Source: CAD feature listing. Evaluate the final solid. Frame: model axes, mm. Face numbers are marked on the shaded views. A direction names the side the tool comes from. Give positions to 0.01 mm unless a question says otherwise; leave off trailing zeros. Order: outer loops, then holes, each group sorted by start corner. A loop starts at its lowest first (then second) coordinate and runs counter-clockwise, first axis right, second up. Notation, with made-up numbers: M 28.25,64.25 L 32.25,64.25 A32 ccw 32.25,99.25 Z; hole C 1.25,15.25 d2. An arc over 180 degrees is marked long. Use CSV: the item, a comma, the result in double quotes. Start each with the question number.
Item 1: Section query A-A on y = 60. Count the separate pieces of the cut face and the enclosed holes in it, and give its area (3 significant figures).
Item 2: Section query B-B on z = 3.5. Return loops of the section in (x, y), and give its area (3 significant figures).
Item 3: First-contact query: pin 1 (10 mm diameter, centred on x = -232.5, z = 23, fed in from -Y); pin 2 (17 mm diameter, centred on x = -6.5, z = 10, fed in from -Y). Flat tips, straight axial feed; report the tip coordinate or a pass-through.
Item 4: Pull-direction query (Z, two-part tool) for the marked faces 3, 4, 5 and 6; classes: +Z half, -Z half, draft (parallel to the pull), parting line (faces both ways), or undercut.
Item 5: Ray query, probe 1 along X at (y, z) = (44.5, 28); probe 2 along X at (y, z) = (75, 3.5); probe 3 along X at (y, z) = (66, 84). Return the intervals inside material, ascending. Write a range as from..to.
Item 6: Access query for the marked faces 1 and 2. Directions: +Z, -Z, +X, -X, +Y, -Y. A direction counts if a zero-diameter tool reaches every point of the face in a straight line with its end or side. Return the directions, or none.
Item 7: Section query D-D on x = -157. Return loops of the section in (y, z).
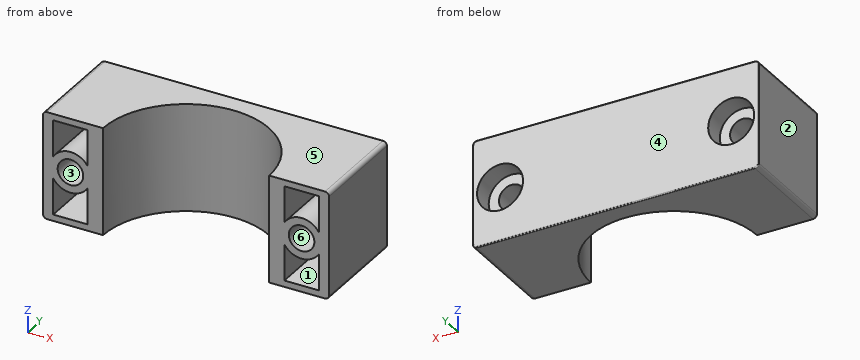
Autodesk Inventor part; units mm, degrees
ref_plane "YZ Plane" through (0, 0, 0) normal (1, 0, 0) x (0, 1, 0)
ref_plane "XZ Plane" through (0, 0, 0) normal (0, 1, 0) x (-1, 0, 0)
ref_plane "XY Plane" through (0, 0, 0) normal (0, 0, 1) x (1, 0, 0)
sketch "Sketch2" plane through (0, 0, 0) normal (0, 1, 0) x (-1, 0, 0)
  line L0 (-15.2041, -8.8425) -> (269.2759, -8.8425)
  line L1 (269.2759, -8.8425) -> (269.2759, 97.8375)
  line L2 (269.2759, 97.8375) -> (-15.2041, 97.8375)
  line L3 (-15.2041, 97.8375) -> (-15.2041, -8.8425)
  point P0 (0, 0)
  dimension "d5" = 284.48
  dimension "d6" = 106.68
  dimension "d7" = 284.48
  dimension "d8" = 106.68
extrude "Extrusion1" add sketch "Sketch2" along normal blind 101.6
sketch "Sketch3" plane through (15.2041, 0, -8.8425) normal (0, 0, -1) x (-1, 0, 0)
  line L0 (0, 0) -> (284.48, 0)
  arc A0 (224.79, 0) -> (59.69, 0) centre (142.24, 0) ccw
  line L1 (59.69, 0) -> (224.79, 0)
  point P0 (15.2041, 0)
extrude "Extrusion2" cut sketch "Sketch3" against normal blind 127
sketch "Sketch4" plane through (0, 0, 0) normal (0, -1, 0) x (1, 0, 0)
  line L0 (-209.5859, -8.8425) -> (-209.5859, 97.8375)
  line L1 (-269.2759, 97.8375) -> (-209.5859, 97.8375)
  line L2 (-269.2759, -8.8425) -> (-269.2759, 97.8375)
  line L3 (-209.5859, -8.8425) -> (-269.2759, -8.8425)
  line L4 (-44.4859, 97.8375) -> (15.2041, 97.8375)
  line L5 (-44.4859, 97.8375) -> (-44.4859, -8.8425)
  line L6 (15.2041, -8.8425) -> (-44.4859, -8.8425)
  line L7 (15.2041, 97.8375) -> (15.2041, -8.8425)
  line L8 (-44.4859, 97.8375) -> (15.2041, 97.8375)
  line L9 (-241.3709, 97.8375) -> (-241.3709, 91.4875) construction
  line L10 (-209.5859, 77.888) -> (-224.8259, 77.888) construction
  line L11 (-269.2759, 47.5596) -> (-259.1159, 47.5596) construction
  line L12 (-239.4309, -8.8425) -> (-239.4309, -2.4925) construction
  line L13 (-259.1159, -2.4925) -> (-259.1159, 91.4875)
  line L14 (-259.1159, 91.4875) -> (-224.8259, 91.4875)
  line L15 (-224.8259, 91.4875) -> (-224.8259, -2.4925)
  line L16 (-224.8259, -2.4925) -> (-259.1159, -2.4925)
  point P0 (0, 0)
  dimension "d15" = 6.35
  dimension "d16" = 15.24
  dimension "d17" = 10.16
  dimension "d18" = 6.35
extrude "Extrusion3" cut sketch "Sketch4" against normal blind 76.2 contours L13 L14 L15 L16
sketch "Sketch5" plane through (0, 76.2, 0) normal (0, -1, 0) x (1, 0, 0)
  line L0 (-259.1159, 91.4875) -> (-224.8259, 91.4875)
  line L1 (-259.1159, -2.4925) -> (-259.1159, 91.4875)
  line L2 (-224.8259, -2.4925) -> (-259.1159, -2.4925)
  line L3 (-224.8259, 91.4875) -> (-224.8259, -2.4925)
  line L4 (-259.1159, 44.4975) -> (-224.8259, 44.4975) construction
  line L5 (-241.9709, 91.4875) -> (-241.9709, 84.1907) construction
  line L6 (-241.9709, 84.1907) -> (-241.9709, 84.1907) construction
  line L7 (-241.9709, 84.1907) -> (-241.9709, -2.4925) construction
  circle A0 centre (-241.9709, 44.4975) radius 20.32
  point P0 (0, 0)
  dimension "d21" = 40.64
  dimension "d22" = 0
extrude "Extrusion4" add sketch "Sketch5" along normal blind 76.2 contours A0 L3 L1 | L1 A0 | A0 L3
sketch "Sketch6" plane through (0, 0, 0) normal (0, -1, 0) x (1, 0, 0)
  arc A0 (-259.1159, 33.5911) -> (-224.8259, 33.5911) centre (-241.9709, 44.4975) ccw
  circle A1 centre (-241.9709, 44.4975) radius 12.7
  point P0 (0, 0)
  dimension "d25" = 25.4
extrude "Extrusion5" cut sketch "Sketch6" against normal blind 101.6
sketch "Sketch7" plane through (0, 101.6, 0) normal (0, 1, 0) x (1, 0, 0)
  circle A0 centre (-241.9709, -44.4975) radius 12.7
  circle A1 centre (-241.9709, -44.4975) radius 22.86
  point P0 (0, 0)
  dimension "d29" = 45.72
extrude "Extrusion6" cut sketch "Sketch7" against normal blind 20.32
sketch "Sketch8" plane through (0, 0, 0) normal (0, -1, 0) x (1, 0, 0)
  line L0 (-44.4859, 97.8375) -> (-44.4859, -8.8425)
  line L1 (15.2041, -8.8425) -> (-44.4859, -8.8425)
  line L2 (15.2041, 97.8375) -> (15.2041, -8.8425)
  line L3 (-44.4859, 97.8375) -> (15.2041, 97.8375)
  line L4 (-44.4859, 51.8911) -> (-29.2459, 51.8911) construction
  line L5 (15.2041, 49.6514) -> (5.0441, 49.6514) construction
  line L6 (-16.6435, -8.8425) -> (-16.6435, -2.4925) construction
  line L7 (-14.6409, 97.8375) -> (-14.6409, 91.4875) construction
  line L8 (5.0441, 91.4875) -> (-29.2459, 91.4875)
  line L9 (-29.2459, 91.4875) -> (-29.2459, -2.4925)
  line L10 (-29.2459, -2.4925) -> (5.0441, -2.4925)
  line L11 (5.0441, -2.4925) -> (5.0441, 91.4875)
  point P0 (0, 0)
  dimension "d32" = 15.24
  dimension "d33" = 10.16
  dimension "d34" = 6.35
  dimension "d35" = 6.35
extrude "Extrusion7" cut sketch "Sketch8" against normal blind 76.2 contours L11 L10 L9 L8
sketch "Sketch9" plane through (0, 76.2, 0) normal (0, -1, 0) x (1, 0, 0)
  line L0 (-29.2459, 91.4875) -> (5.0441, 91.4875)
  line L1 (-29.2459, -2.4925) -> (-29.2459, 91.4875)
  line L2 (5.0441, -2.4925) -> (-29.2459, -2.4925)
  line L3 (-12.1009, -2.4925) -> (-12.1009, 91.4875) construction
  line L4 (-29.2459, 44.4975) -> (0, 44.4975) construction
  circle A0 centre (-12.1009, 44.4975) radius 20.32
  point P0 (0, 0)
  dimension "d38" = 40.64
extrude "Extrusion8" add sketch "Sketch9" along normal blind 76.2
sketch "Sketch10" plane through (0, 0, 0) normal (0, -1, 0) x (1, 0, 0)
  arc A0 (-29.2459, 33.5911) -> (5.0441, 33.5911) centre (-12.1009, 44.4975) ccw
  circle A1 centre (-12.1009, 44.4975) radius 12.7
  point P0 (0, 0)
  dimension "d41" = 25.4
extrude "Extrusion9" cut sketch "Sketch10" against normal blind 101.6
sketch "Sketch11" plane through (0, 101.6, 0) normal (0, 1, 0) x (1, 0, 0)
  circle A0 centre (-12.1009, -44.4975) radius 12.7
  circle A1 centre (-12.1009, -44.4975) radius 22.86
  point P0 (0, 0)
  dimension "d44" = 45.72
extrude "Extrusion10" cut sketch "Sketch11" against normal blind 20.32
fillet "Fillet1" radius 4 4 edges at (15.2041, 50.8, 97.8375) (15.2041, 50.8, -8.8425) (-269.2759, 50.8, 97.8375) (-269.2759, 50.8, -8.8425)
fillet "Fillet2" radius 1 8 edges at (14.0325, 101.6, 96.666) (15.2041, 101.6, 44.4975) (14.0325, 101.6, -7.6709) (-127.0359, 101.6, -8.8425) (-268.1044, 101.6, -7.6709) (-269.2759, 101.6, 44.4975) (-268.1044, 101.6, 96.666) (-127.0359, 101.6, 97.8375)
properties part number "CIM mount" material "Polypropylene"
Verdict:
1,separate pieces,"2"
1,enclosed holes,"6"
1,area,"13,200 mm2"
2,outline,"M -269.28,0 L -259.12,0 L -259.12,76.2 L -224.83,76.2 L -224.83,0 L -209.59,0 A82.55 cw -44.49,0 L -29.25,0 L -29.25,76.2 L 5.04,76.2 L 5.04,0 L 15.2,0 L 15.2,100.6 A1 ccw 14.2,101.6 L -268.28,101.6 A1 ccw -269.28,100.6 Z"
2,area,"13,000 mm2"
3,pin 1,"y = 0"
3,pin 2,"y = 76.2"
4,face 3,"undercut"
4,face 4,"draft"
4,face 5,"+Z half"
4,face 6,"undercut"
5,probe 1,"-269.28..-259.12, -253.83..-230.11, -224.83..-196.56, -57.51..-29.25, -23.96..-0.24, 5.04..15.2"
5,probe 2,"-269.28..-259.12, -224.83..-161.53, -92.55..-29.25, 5.04..15.2"
5,probe 3,"-269.28..-259.12, -224.83..-176.62, -77.45..-29.25, 5.04..15.2"
6,face 1,"-Y"
6,face 2,"+Z, -Z, -X, +Y, -Y"
7,outline,"M 76.92,-8.84 L 100.6,-8.84 A1 ccw 101.6,-7.84 L 101.6,96.84 A1 ccw 100.6,97.84 L 76.92,97.84 Z"
